For this review, take the finished solid that the model builds, in its own axes (mm). A direction names the side the tool comes from. Coordinates: 2 decimals unless noted, no trailing zeros. Loops run counter-clockwise (first coordinate to the right, second up) from the corner with the lowest first, then second, coordinate; pieces in that order, holes last.
1. Take a section at C-C, the plane z = 9.5. State the section outline as (x, y) points, then the cut area to 3 significant figures.
2. Take a section at A-A, the plane y = 9.5. State the section outline as (x, z) points, then the cut area to 3 significant figures.
3. Mouldability with a two-part tool opening along Y and no side actions: class faces 1 (the face through (-0.242, 35.495, 21.486)), 2 (the face through (0, 15, 23.5)), 3 (the face through (-8.196, 36.289, -21.472)) as pulls with the +Y half, pulls with the -Y half, needs draft (parallel to the pull), parting line crosses it, or undercut.
4. Clearance check with flat-ended pins moving along their axes: P1, Ø3, axis at x = 0, z = -9.5, coming from the +Y side; P2, Ø3, axis at x = -7.5, z = -6.5, coming from the +Y side; P3, Ø2, axis at x = -1, y = 21, coming from the -Z side; P4, Ø8, axis at x = -3, y = 26, coming from the -Z side. State where each tip first meets the part, or that it passes through.
5. To check wall thickness, follow probe 1 along Z at (x, y) = (0, 1.7); probe 2 along X at (y, z) = (30, -22); probe 3 along X at (y, z) = (23.5, -20.85). State the ranges of each line that lie inside material, in increasing order.
6. Take a section at B-B, the plane x = 0. Count the separate pieces of the cut face and the enclosed holes in it, then the cut area to 3 significant figures.
7. Machinability: for faces 4 (the face through (-0.526, 1.521, -11.169)), 5 (the face through (0, 20, -19.5)), 6 (the face through (0, 20, -21.5)), which of the approach directions +Z, -Z, +X, -X, +Y, -Y give a long, thin tool a straight path to every point of the face, cutting with its end or side? Answer none if there is none.
8. Take a section at D-D, the plane z = -16.5. State the section outline as (x, y) points, then the cut area to 3 significant figures.
Autodesk Inventor part; units mm, degrees
ref_plane "YZ Plane" through (0, 0, 0) normal (1, 0, 0) x (0, 1, 0)
ref_plane "XZ Plane" through (0, 0, 0) normal (0, 1, 0) x (-1, 0, 0)
ref_plane "XY Plane" through (0, 0, 0) normal (0, 0, 1) x (1, 0, 0)
sketch "Sketch1" plane through (0, 0, 0) normal (0, 1, 0) x (-1, 0, 0)
  line L0 (14, 0) -> (-14, 0)
  line L1 (0, -32.9) -> (0, 32.9)
  line L2 (10, 23.5) -> (-10, 23.5)
  line L3 (-10, 23.5) -> (-10, -23.5)
  line L4 (-10, -23.5) -> (10, -23.5)
  line L5 (10, -23.5) -> (10, 23.5)
  point P0 (0, 0)
  dimension "d0" = 47
  dimension "d1" = 20
extrude "Extrusion1" add sketch "Sketch1" along normal blind 3
sketch "Sketch2" plane through (0, 3, 0) normal (0, 1, 0) x (1, 0, 0)
  line L0 (-10, -23.5) -> (10, -23.5)
  line L1 (10, -23.5) -> (10, 23.5)
  line L2 (10, 23.5) -> (-10, 23.5)
  line L3 (-10, 23.5) -> (-10, -23.5)
  line L4 (-10, -23.5) -> (10, -23.5)
  line L5 (10, -23.5) -> (10, -19.5)
  line L6 (10, -19.5) -> (-10, -19.5)
  line L7 (-10, -19.5) -> (-10, -23.5)
  line L8 (-10, 19.5) -> (10, 19.5)
  line L9 (10, 19.5) -> (10, 23.5)
  line L10 (10, 23.5) -> (-10, 23.5)
  line L11 (-10, 23.5) -> (-10, 19.5)
  line L12 (-10, -23.5) -> (10, -23.5)
  line L13 (-10, 23.5) -> (-10, -23.5)
  line L14 (10, -23.5) -> (10, 23.5)
  line L15 (10, 23.5) -> (-10, 23.5)
  point P0 (0, 0)
  dimension "d4" = 4
  dimension "d5" = 4
extrude "Extrusion2" add sketch "Sketch2" along normal blind 35 contours L3 L6 L1 L0 | L3 L2 L1 L8
sketch "Sketch3" plane through (-10, 0, 23.5) normal (0, 0, 1) x (1, 0, 0)
  point P0 (10, 0)
sketch "Sketch4" plane through (-10, 0, 23.5) normal (0, 0, 1) x (1, 0, 0)
  line L0 (0, 0) -> (20, 0)
  line L1 (20, 0) -> (20, 38)
  line L2 (0, 38) -> (20, 38)
  line L3 (0, 0) -> (0, 38)
  point P0 (10, 0)
  point P1 (10, 30)
  dimension "d8" = 10
  dimension "d9" = 8
hole "Hole1" at (0, 30, 23.5) direction (0, 0, -1) diameter 11 depth 43
fillet "Fillet1" radius 6 4 edges at (10, 38, -21.5) (-10, 38, -21.5) (10, 38, 21.5) (-10, 38, 21.5)
sketch "Sketch8" plane through (0, 0, 0) normal (0, -1, 0) x (1, 0, 0)
  line L0 (-10, 23.5) -> (10, 23.5)
  line L1 (-10, -23.5) -> (-10, 23.5)
  line L2 (10, -23.5) -> (-10, -23.5)
  line L3 (10, 23.5) -> (10, -23.5)
  line L4 (-14, 0) -> (14, 0)
  line L5 (0, -32.9) -> (0, 32.9)
  line L6 (10, -19.5) -> (-10, -19.5)
  line L7 (-10, 19.5) -> (10, 19.5)
  point P0 (0, 0)
  point P1 (0, -9.5)
  point P2 (0, 9.5)
  dimension "d37" = 10
  dimension "d38" = 10
  dimension "d75" = 19
hole "Hole3" at (0, 0, 9.5) at (0, 0, -9.5) direction (0, 1, 0) diameter 3.5 end through all
sketch "Sketch10" plane through (10, 0, -23.5) normal (0, 0, -1) x (-1, 0, 0)
  arc A0 (20, 32) -> (14, 38) centre (14, 32) ccw
  line L0 (6, 38) -> (14, 38)
  arc A1 (6, 38) -> (0, 32) centre (6, 32) ccw
  line L1 (0, 0) -> (0, 32)
  line L2 (0, 0) -> (20, 0)
  line L3 (20, 0) -> (20, 32)
  circle A2 centre (10, 30) radius 5.5
  circle A3 centre (10, 30) radius 3.75
  circle A4 centre (10, 16) radius 2.5
  line L4 (-6.7241, 13.5) -> (37.2046, 13.5) construction
  line L5 (6.25, 30) -> (7.5505, 15.5)
  line L6 (13.75, 30) -> (12.4495, 15.5)
  point P0 (10, 0)
  dimension "d47" = 16.5
  dimension "d48" = 7.5
  dimension "d49" = 5
  dimension "d50" = 10
  dimension "d51" = 2
  dimension "d52" = 2
  dimension "d53" = 8
  dimension "d54" = 8
extrude "Extrusion4" cut sketch "Sketch10" against normal blind 2 contours L5 A3 L6 A2 | A2 L6 A4 L5 | L5 A3 L6 | A4 L6 L5 picked at (9.6017, 25.1271)
sketch "Sketch11" plane through (10, 0, -21.5) normal (0, 0, -1) x (-1, 0, 0)
  line L0 (7.5505, 15.5) -> (6.25, 30)
  arc A0 (7.5505, 15.5) -> (12.4495, 15.5) centre (10, 16) ccw
  line L1 (13.75, 30) -> (12.4495, 15.5)
  arc A1 (13.75, 30) -> (6.25, 30) centre (10, 30) ccw
  point P0 (10, 0)
hole "Hole4" at (0, 30, -21.5) direction (0, 0, 1) diameter 7.5 depth 41
sketch "Sketch12" plane through (10, 0, -21.5) normal (0, 0, -1) x (-1, 0, 0)
  arc A0 (6.3099, 29.3327) -> (13.6901, 29.3327) centre (10, 30) ccw
  line L0 (7.5505, 15.5) -> (6.3099, 29.3327)
  arc A1 (7.5505, 15.5) -> (12.4495, 15.5) centre (10, 16) ccw
  line L1 (13.6901, 29.3327) -> (12.4495, 15.5)
  line L2 (0, 0) -> (0, 32)
  point P0 (10, 0)
  point P1 (10, 23.5)
  dimension "d64" = 6.5
  dimension "d65" = 10
hole "Hole5" at (0, 23.5, -21.5) direction (0, 0, 1) diameter 2.5 depth 41
fillet "Fillet2" radius 1 1 edges at (0, 35.5, 19.5)
fillet "Fillet3" radius 1 1 edges at (0, 35.5, 23.5)
properties part number "new_femur"
Results list:
1. outline: (-10, 0) - (-1.75, 0) - (-1.75, 3) - (-10, 3) - close; (1.75, 0) - (10, 0) - (10, 3) - (1.75, 3) - close
1. area: 49.5 mm2
2. outline: (-10, -23.5) - (10, -23.5) - (10, -19.5) - (-10, -19.5) - close; (-10, 19.5) - (10, 19.5) - (10, 23.5) - (-10, 23.5) - close
2. area: 160 mm2
3. face 1: undercut
3. face 2: needs draft
3. face 3: pulls with the +Y half
4. P1: passes through
4. P2: stops at y = 3
4. P3: stops at z = -21.5
4. P4: stops at z = -23.5
5. probe 1: z = -23.5 to -11.25, -7.75 to 7.75, 11.25 to 23.5
5. probe 2: x = -10 to -3.75, 3.75 to 10
5. probe 3: x = -10 to -1.25, 1.25 to 10
6. separate pieces: 6
6. enclosed holes: 0
6. area: 295 mm2
7. face 4: +Y, -Y
7. face 5: +X, -X, +Y
7. face 6: -Z
8. outline: (-10, 0) - (10, 0) - (10, 3) - (-10, 3) - close
8. area: 60.0 mm2
